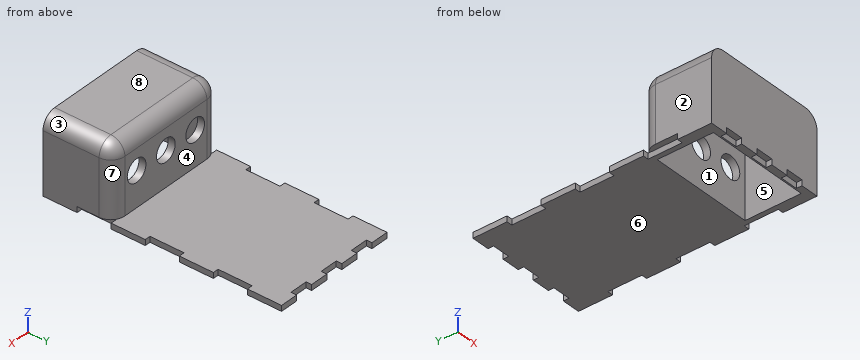
from build123d import *

# Parameters (mm, degrees)
BUITENAFMETING_RECHTHOEK_W  = 90
BUITENAFMETING_RECHTHOEK_H  = 170
PLAAT_DEPTH                 = 4
TAND_HOR_W                  = 12.857142857
TAND_HOR_H                  = 4
TAND_BOVEN_DEPTH            = 193.395426141
TANDEN_PATROON_BOVEN_COUNT  = 3
TANDEN_PATROON_BOVEN_PITCH  = 25.714285714
TAND_VER_W                  = 4
TAND_VER_H                  = 24.285714285
TAND_LINKS_DEPTH            = 193.395426141
TANDEN_PATROON_LINKS_COUNT  = 3
TANDEN_PATROON_LINKS_PITCH  = 48.571428571
TAND_O_W                    = 12.857142857
TAND_O_H                    = 4
TAND_ONDER_DEPTH            = 193.395426141
TANDEN_PATROON_ONDER_COUNT  = 3
TANDEN_PATROON_ONDER_PITCH  = 25.714285714
TAND_R_W                    = 4
TAND_R_H                    = 24.285714285
TAND_RECHTS_DEPTH           = 193.395426141
TANDEN_PATROON_RECHTS_COUNT = 3
TANDEN_PATROON_RECHTS_PITCH = 48.571428571
SKETCH1_W                   = 90
SKETCH1_H                   = 50
BOSS_EXTRUDE1_DEPTH         = 50
SKETCH2_W                   = 75
SKETCH2_H                   = 40
CUT_EXTRUDE1_DEPTH          = 50
SKETCH3_R                   = 8
CUT_EXTRUDE3_DEPTH          = 24
FILLET1_R                   = 10


with BuildPart() as part:
    # Buitenafmeting Rechthoek → Plaat (new body)
    with BuildSketch(Plane.XY):
        with Locations((45, 85)):
            Rectangle(BUITENAFMETING_RECHTHOEK_W, BUITENAFMETING_RECHTHOEK_H)
    extrude(amount=-PLAAT_DEPTH)

    # Tand Hor → Tand Boven (cut, through all)
    with BuildSketch(Plane.XY):
        with Locations((19.285714286, 168)):
            Rectangle(TAND_HOR_W, TAND_HOR_H)
    tand_boven = extrude(amount=-TAND_BOVEN_DEPTH, mode=Mode.SUBTRACT)

    # Tanden Patroon Boven: Tand Boven ×3
    with Locations(*[(i * TANDEN_PATROON_BOVEN_PITCH, 0, 0) for i in range(1, TANDEN_PATROON_BOVEN_COUNT)]):
        add(tand_boven, mode=Mode.SUBTRACT)

    # Tand Ver → Tand Links (cut, through all)
    with BuildSketch(Plane.XY):
        with Locations((2, 133.571428572)):
            Rectangle(TAND_VER_W, TAND_VER_H)
    tand_links = extrude(amount=-TAND_LINKS_DEPTH, mode=Mode.SUBTRACT)

    # Tanden Patroon Links: Tand Links ×3
    with Locations(*[(0, -i * TANDEN_PATROON_LINKS_PITCH, 0) for i in range(1, TANDEN_PATROON_LINKS_COUNT)]):
        add(tand_links, mode=Mode.SUBTRACT)

    # Tand O → Tand Onder (cut, through all)
    with BuildSketch(Plane.XY):
        with Locations((19.285714286, 2)):
            Rectangle(TAND_O_W, TAND_O_H)
    tand_onder = extrude(amount=-TAND_ONDER_DEPTH, mode=Mode.SUBTRACT)

    # Tanden Patroon Onder: Tand Onder ×3
    with Locations(*[(i * TANDEN_PATROON_ONDER_PITCH, 0, 0) for i in range(1, TANDEN_PATROON_ONDER_COUNT)]):
        add(tand_onder, mode=Mode.SUBTRACT)

    # Tand R → Tand Rechts (cut, through all)
    with BuildSketch(Plane.XY):
        with Locations((88, 133.571428572)):
            Rectangle(TAND_R_W, TAND_R_H)
    tand_rechts = extrude(amount=-TAND_RECHTS_DEPTH, mode=Mode.SUBTRACT)

    # Tanden Patroon Rechts: Tand Rechts ×3
    with Locations(*[(0, -i * TANDEN_PATROON_RECHTS_PITCH, 0) for i in range(1, TANDEN_PATROON_RECHTS_COUNT)]):
        add(tand_rechts, mode=Mode.SUBTRACT)

    # Sketch1 → Boss-Extrude1 (add)
    with BuildSketch(Plane.XY):
        with Locations((45, 25)):
            Rectangle(SKETCH1_W, SKETCH1_H)
    extrude(amount=BOSS_EXTRUDE1_DEPTH)

    # Sketch2 → Cut-Extrude1 (cut)
    with BuildSketch(Plane(origin=(0, 0, -4), x_dir=(-1, 0, 0), z_dir=(0, 0, -1))):
        with Locations((-45, 25)):
            Rectangle(SKETCH2_W, SKETCH2_H)
    extrude(amount=-CUT_EXTRUDE1_DEPTH, mode=Mode.SUBTRACT)

    # Sketch3 → Cut-Extrude3 (cut)
    with BuildSketch(Plane(origin=(0, 50, 0), x_dir=(1, 0, 0), z_dir=(0, 1, 0))):
        with Locations(Location((45, -25, 0), (0, 0, 270))):
            Circle(SKETCH3_R)
        with Locations(Location((70, -25, 0), (0, 0, 270))):
            Circle(SKETCH3_R)
        with Locations(Location((20, -25, 0), (0, 0, 270))):
            Circle(SKETCH3_R)
    extrude(amount=-CUT_EXTRUDE3_DEPTH, mode=Mode.SUBTRACT)

    # Fillet1
    # the kernel refuses this fillet: 10 mm, written as the material it takes off along each edge
    with BuildSketch(Plane(origin=(10, 40, 40), x_dir=(0, 0, 1), z_dir=(0, 1, 0))) as fillet1_piece_1_section:
        Polygon((0, 0), (FILLET1_R * 1.02, 0), (FILLET1_R * 1.02, -FILLET1_R * 1.02), (0, -FILLET1_R * 1.02), align=None)
    fillet1_piece_1 = extrude(amount=FILLET1_R * 1.02, mode=Mode.PRIVATE)
    fillet1_piece_1 = fillet1_piece_1 - Plane(origin=(10, 40, 40), x_dir=(0.7071067811865475, 0, -0.7071067811865475), z_dir=(0, 1, 0)) * Sphere(FILLET1_R, mode=Mode.PRIVATE)
    add(fillet1_piece_1, mode=Mode.SUBTRACT)
    with BuildSketch(Plane(origin=(80, 40, 40), x_dir=(1, 0, 0), z_dir=(0, 1, 0))) as fillet1_piece_2_section:
        Polygon((0, 0), (FILLET1_R * 1.02, 0), (FILLET1_R * 1.02, -FILLET1_R * 1.02), (0, -FILLET1_R * 1.02), align=None)
    fillet1_piece_2 = extrude(amount=FILLET1_R * 1.02, mode=Mode.PRIVATE)
    fillet1_piece_2 = fillet1_piece_2 - Plane(origin=(80, 40, 40), x_dir=(-0.7071067811865475, 0, -0.7071067811865475), z_dir=(0, 1, 0)) * Sphere(FILLET1_R, mode=Mode.PRIVATE)
    add(fillet1_piece_2, mode=Mode.SUBTRACT)
    with BuildSketch(Plane(origin=(0, 50, 0), x_dir=(0, -1, 0), z_dir=(0, 0, 1))) as fillet1_piece_3:
        with BuildLine():
            CenterArc((FILLET1_R, FILLET1_R), FILLET1_R, 180, 90)
            Line((0, FILLET1_R), (0, 0))
            Line((0, 0), (FILLET1_R, 0))
        make_face()
    extrude(amount=40, mode=Mode.SUBTRACT)
    with BuildSketch(Plane(origin=(90, 50, 0), x_dir=(0, -1, 0), z_dir=(0, 0, 1))) as fillet1_piece_4:
        with BuildLine():
            CenterArc((FILLET1_R, -FILLET1_R), FILLET1_R, 90, 90)
            Line((0, -FILLET1_R), (0, 0))
            Line((0, 0), (FILLET1_R, 0))
        make_face()
    extrude(amount=40, mode=Mode.SUBTRACT)
    with BuildSketch(Plane(origin=(0, 40, 50), x_dir=(1, 0, 0), z_dir=(0, -1, 0))) as fillet1_piece_5:
        with BuildLine():
            CenterArc((FILLET1_R, -FILLET1_R), FILLET1_R, 90, 90)
            Line((0, -FILLET1_R), (0, 0))
            Line((0, 0), (FILLET1_R, 0))
        make_face()
    extrude(amount=65, mode=Mode.SUBTRACT)
    with BuildSketch(Plane(origin=(90, -25, 50), x_dir=(0, 0, -1), z_dir=(0, 1, 0))) as fillet1_piece_6:
        with BuildLine():
            CenterArc((FILLET1_R, FILLET1_R), FILLET1_R, 180, 90)
            Line((0, FILLET1_R), (0, 0))
            Line((0, 0), (FILLET1_R, 0))
        make_face()
    extrude(amount=65, mode=Mode.SUBTRACT)
    with BuildSketch(Plane(origin=(80, 50, 50), x_dir=(0, -1, 0), z_dir=(-1, 0, 0))) as fillet1_piece_7:
        with BuildLine():
            CenterArc((FILLET1_R, -FILLET1_R), FILLET1_R, 90, 90)
            Line((0, -FILLET1_R), (0, 0))
            Line((0, 0), (FILLET1_R, 0))
        make_face()
    extrude(amount=70, mode=Mode.SUBTRACT)


solid = part.part
Check sheet for the modelled part. Datum: model origin and axes. Units: mm. Face numbers are marked on the shaded views. A direction names the side the tool comes from. Give positions to 0.01 mm unless a question says otherwise; leave off trailing zeros. Write each loop counter-clockwise with the first axis right and the second up, starting at its lowest first coordinate (ties: lowest second). Pieces come first, ordered by that corner, then holes. Notation, with made-up numbers: (11.25, -24) -> (50.25, -24) arc R18 ccw to (50.25, -20) -> close; hole circle Ø5 at (74, 64.5). An arc over 180 degrees is marked (long way). One line per item, written item: value. Start each with the question number.
Item 1: Section check A-A on z = 25. Record the cut outline in (x, y), then the cut area to 3 significant figures.
Item 2: Section check C-C on z = 42. Record the cut outline in (x, y).
Item 3: Draft check along X on the marked faces 1, 2 and 3. Enter one of: +X half, -X half, draft (parallel to the pull), parting line (faces both ways), or undercut.
Item 4: Section check D-D on y = 15.5. Record the cut outline in (x, z).
Item 5: Section check B-B on x = 45. Record the cut outline in (y, z), then the cut area to 3 significant figures.
Item 6: Tool access check on the marked faces 4, 5, 6, 7 and 8. Record the directions out of +Z, -Z, +X, -X, +Y, -Y that give a thin tool (end or side, any length) a straight path to the whole face; none if there is none.
Item 7: Material ranges on probe 1 along X at (y, z) = (48, 25); probe 2 along Y at (x, z) = (77, 31.5); probe 3 along X at (y, z) = (23.5, 15.5), recorded low to high. Write a range as from..to.
Item 8: Gauge pin test, flat ends, axial feed: pin 1 (8 mm diameter, centred on x = 13, y = 38, fed in from -Z); pin 2 (2 mm diameter, centred on x = 78.5, z = 12.5, fed in from +Y); pin 3 (2 mm diameter, centred on y = 89.5, z = -2, fed in from -X). Record the tip position at first contact, or that the pin passes through.
Results list:
1. outline: (0, 0) -> (90, 0) -> (90, 40) arc R10 ccw to (80, 50) -> (78, 50) -> (78, 45) -> (82.5, 45) -> (82.5, 5) -> (7.5, 5) -> (7.5, 45) -> (12, 45) -> (12, 50) -> (10, 50) arc R10 ccw to (0, 40) -> close; (28, 45) -> (37, 45) -> (37, 50) -> (28, 50) -> close; (53, 45) -> (62, 45) -> (62, 50) -> (53, 50) -> close
1. area: 1,220 mm²
2. outline: (0.2, 0) -> (89.8, 0) -> (89.8, 40) arc R9.8 ccw to (80, 49.8) -> (10, 49.8) arc R9.8 ccw to (0.2, 40) -> close; hole (7.5, 5) -> (82.5, 5) -> (82.5, 45) -> (7.5, 45) -> close
3. face 1: undercut
3. face 2: -X half
3. face 3: +X half
4. outline: (0, -4) -> (7.5, -4) -> (7.5, 46) -> (82.5, 46) -> (82.5, -4) -> (90, -4) -> (90, 40) arc R10 ccw to (80, 50) -> (10, 50) arc R10 ccw to (0, 40) -> close
5. outline: (0, 0) -> (4, 0) -> (4, -4) -> (5, -4) -> (5, 46) -> (45, 46) -> (45, 33) -> (50, 33) -> (50, 40) arc R10 ccw to (40, 50) -> (0, 50) -> close; (45, -4) -> (166, -4) -> (166, 0) -> (50, 0) -> (50, 17) -> (45, 17) -> close
5. area: 1,050 mm²
6. face 4: +Z, +X, -X, +Y
6. face 5: -Z
6. face 6: -Z, +X, -X, +Y, -Y
6. face 7: +Z, +X, +Y
6. face 8: +Z, +X, -X, +Y, -Y
7. probe 1: 4..12, 28..37, 53..62, 78..86
7. probe 2: 0..5, 45..50
7. probe 3: 0..7.5, 82.5..90
8. pin 1: z = 46
8. pin 2: y = 50
8. pin 3: x = 4
